from build123d import *

# Parameters (mm, degrees)
EXTRUDE_1_DEPTH     = 1500
SKETCH_2_R          = 5
CUT_EXTRUDE_1_DEPTH = 51
SKETCH_3_R          = 5
CUT_EXTRUDE_2_DEPTH = 51


with BuildPart() as part:
    # Эскиз1 → Вытянуть-Тонкостенный1 (new body)
    with BuildSketch(Plane(origin=(0, 0, 0), x_dir=(0, 0, -1), z_dir=(1, 0, 0))):
        Polygon((50, 0), (0, 0), (0, 50), (4, 50), (4, 4), (50, 4), align=None)
    extrude(amount=EXTRUDE_1_DEPTH)

    # Эскиз2 → Вырез-Вытянуть1 (cut, through all)
    with BuildSketch(Plane.XY):
        with Locations((30, 25)):
            Circle(SKETCH_2_R)
        with Locations((90, 25)):
            Circle(SKETCH_2_R)
        with Locations((150, 25)):
            Circle(SKETCH_2_R)
        with Locations((210, 25)):
            Circle(SKETCH_2_R)
        with Locations((270, 25)):
            Circle(SKETCH_2_R)
        with Locations((330, 25)):
            Circle(SKETCH_2_R)
        with Locations((390, 25)):
            Circle(SKETCH_2_R)
        with Locations((450, 25)):
            Circle(SKETCH_2_R)
        with Locations((510, 25)):
            Circle(SKETCH_2_R)
        with Locations((570, 25)):
            Circle(SKETCH_2_R)
        with Locations((630, 25)):
            Circle(SKETCH_2_R)
        with Locations((690, 25)):
            Circle(SKETCH_2_R)
        with Locations((750, 25)):
            Circle(SKETCH_2_R)
        with Locations((810, 25)):
            Circle(SKETCH_2_R)
        with Locations((870, 25)):
            Circle(SKETCH_2_R)
        with Locations((930, 25)):
            Circle(SKETCH_2_R)
        with Locations((990, 25)):
            Circle(SKETCH_2_R)
        with Locations((1050, 25)):
            Circle(SKETCH_2_R)
        with Locations((1110, 25)):
            Circle(SKETCH_2_R)
        with Locations((1170, 25)):
            Circle(SKETCH_2_R)
        with Locations((1230, 25)):
            Circle(SKETCH_2_R)
        with Locations((1290, 25)):
            Circle(SKETCH_2_R)
        with Locations((1350, 25)):
            Circle(SKETCH_2_R)
        with Locations((1410, 25)):
            Circle(SKETCH_2_R)
        with Locations((1470, 25)):
            Circle(SKETCH_2_R)
    extrude(amount=-CUT_EXTRUDE_1_DEPTH, mode=Mode.SUBTRACT)

    # Эскиз3 → Вырез-Вытянуть2 (cut, through all)
    with BuildSketch(Plane.XZ):
        with Locations((30, -25)):
            Circle(SKETCH_3_R)
        with Locations((90, -25)):
            Circle(SKETCH_3_R)
        with Locations((150, -25)):
            Circle(SKETCH_3_R)
        with Locations((210, -25)):
            Circle(SKETCH_3_R)
        with Locations((270, -25)):
            Circle(SKETCH_3_R)
        with Locations((330, -25)):
            Circle(SKETCH_3_R)
        with Locations((390, -25)):
            Circle(SKETCH_3_R)
        with Locations((450, -25)):
            Circle(SKETCH_3_R)
        with Locations((510, -25)):
            Circle(SKETCH_3_R)
        with Locations((570, -25)):
            Circle(SKETCH_3_R)
        with Locations((630, -25)):
            Circle(SKETCH_3_R)
        with Locations((690, -25)):
            Circle(SKETCH_3_R)
        with Locations((750, -25)):
            Circle(SKETCH_3_R)
        with Locations((810, -25)):
            Circle(SKETCH_3_R)
        with Locations((870, -25)):
            Circle(SKETCH_3_R)
        with Locations((930, -25)):
            Circle(SKETCH_3_R)
        with Locations((990, -25)):
            Circle(SKETCH_3_R)
        with Locations((1050, -25)):
            Circle(SKETCH_3_R)
        with Locations((1110, -25)):
            Circle(SKETCH_3_R)
        with Locations((1170, -25)):
            Circle(SKETCH_3_R)
        with Locations((1230, -25)):
            Circle(SKETCH_3_R)
        with Locations((1290, -25)):
            Circle(SKETCH_3_R)
        with Locations((1350, -25)):
            Circle(SKETCH_3_R)
        with Locations((1410, -25)):
            Circle(SKETCH_3_R)
        with Locations((1470, -25)):
            Circle(SKETCH_3_R)
    extrude(amount=-CUT_EXTRUDE_2_DEPTH, mode=Mode.SUBTRACT)


solid = part.part
Build history of the part. All positions in model axes, mm. A direction names the side the tool comes from. Round coordinates to 2 decimals unless told otherwise and drop trailing zeros. Loops run counter-clockwise (first coordinate to the right, second up) from the corner with the lowest first, then second, coordinate; pieces in that order, holes last. Notation, with made-up numbers: (-4.5, 61.25) -> (39.5, 61.25) arc R16 ccw to (39.5, 87.25) -> close; hole circle Ø8 at (-9, 67). An arc over 180 degrees is marked (long way). Answer in a Markdown table with one row per item.
Item 1: Saw through at C-C (y = 11.5). Write the cut outline in (x, z), and give its area (3 significant figures).
Answers below:
| item | result |
|---|---|
| outline | (0, -4) -> (1500, -4) -> (1500, 0) -> (0, 0) -> close |
| area | 6,000 mm² |
Item 2: Which spindle directions (+Z, -Z, +X, -X, +Y, -Y) get a long thin tool onto all of the face, cutting with end or side? Do faces 1 (the flat face through (0, 3, -14)), 2 (the flat face through (740, 27, -4)). Say none if no direction does.
Answers below:
| item | result |
|---|---|
| face 1 | +Z, -Z, -X, +Y, -Y |
| face 2 | -Z, +X, -X, +Y |
Item 3: Saw through at B-B (z = -42). Write the cut outline in (x, y).
Answers below:
| item | result |
|---|---|
| outline | (0, 0) -> (1500, 0) -> (1500, 4) -> (0, 4) -> close |
Item 4: Pin check, flat tips, straight feed: pin 1 (13 mm diameter, centred on x = 1290, z = -25, fed in from +Y); pin 2 (16 mm diameter, centred on x = 630, z = -25, fed in from -Y); pin 3 (1 mm diameter, centred on x = 472, y = 32, fed in from -Z). Stop position of each tip, or through.
Answers below:
| item | result |
|---|---|
| pin 1 | stops at y = 4 |
| pin 2 | stops at y = 0 |
| pin 3 | stops at z = -4 |
Item 5: Saw through at A-A (x = 1209). Write the cut outline in (y, z), and give its area (3 significant figures).
Answers below:
| item | result |
|---|---|
| outline | (0, -50) -> (4, -50) -> (4, -4) -> (50, -4) -> (50, 0) -> (0, 0) -> close |
| area | 384 mm² |
Item 6: Drill centre lines: L1, parallel to Y at x = 930, z = -2; L2, parallel to Y at x = 1079, z = -9; L3, parallel to Z at x = 160, y = 22.5. Where is each one in solid material? Low to high. Write a range as [from, to].
Answers below:
| item | result |
|---|---|
| L1 | y = [0, 20], [30, 50] |
| L2 | y = [0, 4] |
| L3 | z = [-4, 0] |
